Could you check a few things on this model? Use its own coordinates, in mm. Face numbers are marked on the shaded views. A direction names the side the tool comes from. Give positions to 0.01 mm unless a question says otherwise; leave off trailing zeros. Write each loop counter-clockwise with the first axis right and the second up, starting at its lowest first coordinate (ties: lowest second). Pieces come first, ordered by that corner, then holes. Notation, with made-up numbers: (67, 75.5) - (85, 75.5) arc R26 cw to (85, 91.5) - close; hole circle Ø4 at (-20, -40). An arc over 180 degrees is marked (long way). Use one line per item in the form item = value.
Autodesk Inventor part; units mm, degrees
ref_plane "YZ Plane" through (0, 0, 0) normal (1, 0, 0) x (0, 1, 0)
ref_plane "XZ Plane" through (0, 0, 0) normal (0, 1, 0) x (-1, 0, 0)
ref_plane "XY Plane" through (0, 0, 0) normal (0, 0, 1) x (1, 0, 0)
sketch "Sketch1" plane through (0, 0, 0) normal (0, 0, 1) x (1, 0, 0)
  line L0 (0, 0) -> (100, 0)
  line L1 (100, 0) -> (100, 10)
  line L2 (70, 65) -> (30, 65)
  line L3 (0, 10) -> (0, 0)
  line L4 (0, 10) -> (100, 10)
  line L5 (30, 65) -> (30, 0)
  line L6 (70, 65) -> (70, 0)
  dimension "d0" = 100
  dimension "d1" = 10
extrude "Extrusion1" add sketch "Sketch1" along normal blind 10 contours L5 L4 L6 L0 | L5 L2 L6 L4
sketch "Sketch2" plane through (0, 0, 10) normal (0, 0, 1) x (1, 0, 0)
  line L0 (0, 0) -> (100, 0)
  line L1 (100, 0) -> (100, 10)
  line L2 (100, 10) -> (0, 10)
  line L3 (0, 10) -> (0, 0)
extrude "Extrusion2" add sketch "Sketch2" along normal blind 40
sketch "Sketch3" plane through (0, 0, 10) normal (0, 0, 1) x (1, 0, 0)
  line L0 (70, 65) -> (30, 65)
  line L1 (30, 65) -> (70, 65)
  line L2 (70, 65) -> (70, 50)
  line L3 (70, 0) -> (70, 65)
  line L4 (70, 50) -> (30, 50)
  line L5 (30, 65) -> (30, 0)
  line L6 (30, 50) -> (30, 65)
  point P0 (0, 0)
extrude "Extrusion3" add sketch "Sketch3" along normal blind 45
sketch "Sketch4" plane through (30, 65, 0) normal (0, 1, 0) x (1, 0, 0)
  circle A0 centre (20, -30) radius 12
  point P0 (-30, 0)
extrude "Extrusion4" cut sketch "Sketch4" against normal blind 15
sketch "Sketch5" plane through (0, 0, 10) normal (0, 0, 1) x (1, 0, 0)
  circle A0 centre (50, 30) radius 12
  point P0 (0, 0)
extrude "Extrusion5" cut sketch "Sketch5" against normal blind 10
sketch "Sketch6" plane through (30, 0, 0) normal (0, -1, 0) x (1, 0, 0)
  circle A0 centre (-10, 30) radius 10
  circle A1 centre (20, 30) radius 10
  circle A2 centre (50, 30) radius 10
  line L0 (40, 10) -> (40, 55)
  point P0 (-30, 0)
extrude "Extrusion6" cut sketch "Sketch6" against normal blind 10
properties part number "P3-9"
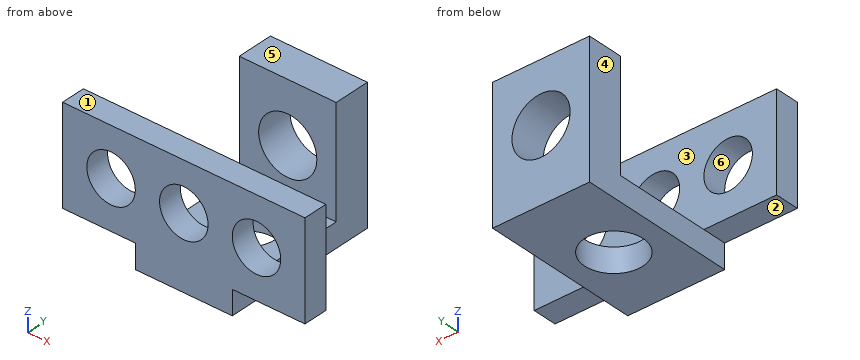
1. Imagine slicing it at D-D, the plane x = 20. List the corners of the cut face in (y, z) for me.
Response values:
outline = (0, 10) - (10, 10) - (10, 20) - (0, 20) - close; (0, 40) - (10, 40) - (10, 50) - (0, 50) - close
2. If we mould it in two halves opening along X, with no side actions, what happens to the marked faces 4, 5 and 6? For each: pulls with the +X half, pulls with the -X half, needs draft (parallel to the pull), parting line crosses it, or undercut.
Response values:
face_4 = pulls with the -X half
face_5 = needs draft
face_6 = undercut
3. Imagine slicing it at C-C, the plane z = 23. List the corners of the cut face in (x, y) for me, and give its area (3 significant figures).
Response values:
outline = (0, 0) - (12.86, 0) - (12.86, 10) - (0, 10) - close; (27.14, 0) - (42.86, 0) - (42.86, 10) - (27.14, 10) - close; (30, 50) - (40.25, 50) - (40.25, 65) - (30, 65) - close; (57.14, 0) - (72.86, 0) - (72.86, 10) - (57.14, 10) - close; (59.75, 50) - (70, 50) - (70, 65) - (59.75, 65) - close; (87.14, 0) - (100, 0) - (100, 10) - (87.14, 10) - close
area = 879 mm²
4. Imagine slicing it at B-B, the plane y = 30. List the corners of the cut face in (x, z) for me, and give its area (3 significant figures).
Response values:
outline = (30, 0) - (38, 0) - (38, 10) - (30, 10) - close; (62, 0) - (70, 0) - (70, 10) - (62, 10) - close
area = 160 mm²
5. Which directions (+Z, -Z, +X, -X, +Y, -Y) give clear straight access to the entire face, cutting with the end or side of a thin tool? Please do the marked faces 1, 2 and 3.
Response values:
face_1 = +Z, +X, -X, -Y
face_2 = -Z, -X, +Y, -Y
face_3 = +Z, +X, -X
6. For pin 1 (16.5 mm diameter, centred on y = 22.5, z = 14.5, fed in from +X); pin 2 (3 mm diameter, centred on x = 18.5, y = 5, fed in from -Z); pin 3 (12 mm diameter, centred on x = 53, z = 25.5, fed in from +Y), each with a flat end and sliding along its axis, tell me the tip position at first contact or that it passes through.
Response values:
pin_1 = 70
pin_2 = 10
pin_3 = 10
7. If I drill on line 1 (Y direction, x = 33.5, z = 24); line 2 (Y direction, x = 50, z = 2.5); line 3 (Z direction, x = 20, y = 6.25), over which ranges is the centre line in solid material (lowest first)? Write a range as from..to.
Response values:
line_1 = 0..10, 50..65
line_2 = 0..18, 42..65
line_3 = 10..20, 40..50
8. Imagine slicing it at A-A, the plane x = 50. List the corners of the cut face in (y, z) for me, and give its area (3 significant figures).
Response values:
outline = (0, 0) - (18, 0) - (18, 10) - (10, 10) - (10, 20) - (0, 20) - close; (0, 40) - (10, 40) - (10, 50) - (0, 50) - close; (42, 0) - (65, 0) - (65, 18) - (50, 18) - (50, 10) - (42, 10) - close; (50, 42) - (65, 42) - (65, 55) - (50, 55) - close
area = 925 mm²
